```python
from build123d import *

# Parameters (mm, degrees)
F1_DEPTH = 10
F2_W     = 10
F2_H     = 18
F3_DEPTH = 10
F4_R     = 5
F5_DEPTH = 10.001
F6_DEPTH = 10.001
F7_R     = 5


with BuildPart() as f1:
    # F0 (on Top) → F1 (new body)
    with BuildSketch(Plane.XY):
        Polygon((65, 40), (0, 40), (-65, 40), (-65, -40), (0, -40), (65, -40), align=None)
    extrude(amount=F1_DEPTH)

    # F2 (on face) → F3 (join)
    with BuildSketch(Plane.XY.offset(10)):
        Polygon((-9, 30), (0, 30), (9, 30), (9, 40), (-9, 40), align=None)
        with Locations((60, 0)):
            Rectangle(F2_W, F2_H)
        Polygon((-55, 9), (-65, 9), (-65, 0), (-65, -9), (-55, -9), align=None)
        Polygon((-9, -40), (9, -40), (9, -30), (0, -30), (-9, -30), align=None)
    extrude(amount=F3_DEPTH)

    # F4 (on face) → F5 (cut, through all)
    with BuildSketch(Plane.XY.offset(10)):
        with Locations((-45, -20)):
            Circle(F4_R)
        with Locations((45, -20)):
            Circle(F4_R)
        with Locations((45, 20)):
            Circle(F4_R)
        with Locations((-45, 20)):
            Circle(F4_R)
    extrude(amount=-F5_DEPTH, mode=Mode.SUBTRACT)

    # F4 (on face) → F6 (cut, through all)
    with BuildSketch(Plane.XY.offset(10)):
        with Locations((-45, -20)):
            Circle(F4_R)
        with Locations((45, -20)):
            Circle(F4_R)
        with Locations((45, 20)):
            Circle(F4_R)
        with Locations((-45, 20)):
            Circle(F4_R)
    extrude(amount=-F6_DEPTH, mode=Mode.SUBTRACT)

    # F7
    f7_edges = [f1.edges().sort_by_distance(p)[0] for p in [
        (-65, -40, 5),
        (65, -40, 5),
        (65, 40, 5),
        (-65, 40, 5),
    ]]
    fillet(f7_edges, radius=F7_R)


solid = f1.part
```
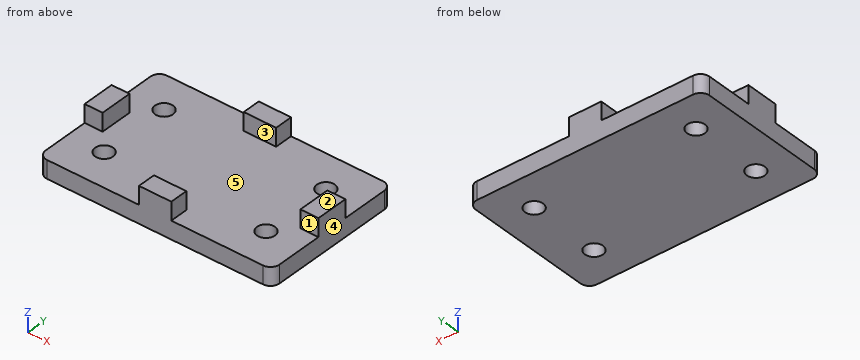
Could you check a few things on this model? Use its own coordinates, in mm. Face numbers are marked on the shaded views. A direction names the side the tool comes from. Round coordinates to 2 decimals unless told otherwise and drop trailing zeros. Write each loop counter-clockwise with the first axis right and the second up, starting at its lowest first coordinate (ties: lowest second). Pieces come first, ordered by that corner, then holes. Notation, with made-up numbers: M 77,-3.75 L 94,-3.75 A18 ccw 94,12.25 Z; hole C -2,62 d6. An arc over 180 degrees is marked long. Write each question's results on one line, items separated by ' | '. Start each with the question number.
1. I'm going to push flat-ended pins straight in: pin 1 Ø8 at (y, z) = (-33.5, 16) entering from -X; pin 2 Ø6 at (x, y) = (45, -20) entering from -Z; pin 3 Ø8 at (x, z) = (61.5, 16.5) entering from +Y; pin 4 Ø4 at (y, z) = (-29, 15.5) entering from +X. Where does each tip first touch, or does it pass through?
2. On a 3-axis mill with a long thin cutter (end or side, diameter ignored), from which of +Z, -Z, +X, -X, +Y, -Y can I reach the whole of each face in a straight line? I mean the marked faces 1 and 2. Say none if no direction works.
3. Imagine slicing it at A-A on y = 20. List the corners of the cut face in (x, z) for me.
4. Thinking about a two-plate mould opening in X: for the marked faces 3, 4 and 5, which applies, +X half, -X half, draft (parallel to the pull), parting line (faces both ways), or undercut?
5. Imagine slicing it at D-D on y = 0.5. List the corners of the cut face in (x, z) for me, and give its area (3 significant figures).
6. I need wall thicknesses on L1, parallel to Y at x = -45.5, z = 3; L2, parallel to Y at x = -42, z = 9.75; L3, parallel to X at y = -4, z = 14.75. Which ranges of each line are inside material? Lowest first, please. Write a range as from..to.
7. Imagine slicing it at B-B on x = 45. List the corners of the cut face in (y, z) for me.
8. Imagine slicing it at C-C on z = 5.5. List the corners of the cut face in (x, y) for me.
Result sheet:
1) pin 1: stops at x = -9 | pin 2: passes through | pin 3: stops at y = 9 | pin 4: stops at x = 9
2) face 1: +Z, +X, -X, -Y | face 2: +Z, +X, -X, +Y, -Y
3) outline: M -65,0 L -50,0 L -50,10 L -65,10 Z; M -40,0 L 40,0 L 40,10 L -40,10 Z; M 50,0 L 65,0 L 65,10 L 50,10 Z
4) face 3: draft | face 4: +X half | face 5: undercut
5) outline: M -65,0 L 65,0 L 65,20 L 55,20 L 55,10 L -55,10 L -55,20 L -65,20 Z | area: 1,500 mm^2
6) L1: y = -40..-24.97, -15.03..15.03, 24.97..40 | L2: y = -40..-24, -16..16, 24..40 | L3: x = -65..-55, 55..65
7) outline: M -40,0 L -25,0 L -25,10 L -40,10 Z; M -15,0 L 15,0 L 15,10 L -15,10 Z; M 25,0 L 40,0 L 40,10 L 25,10 Z
8) outline: M -65,-35 A5 ccw -60,-40 L 60,-40 A5 ccw 65,-35 L 65,35 A5 ccw 60,40 L -60,40 A5 ccw -65,35 Z; hole C -45,-20 d10; hole C -45,20 d10; hole C 45,-20 d10; hole C 45,20 d10
